from build123d import *

# Parameters (mm, degrees)
BOSS_EXTRUDE1_DEPTH      = 15
BOSS_EXTRUDE1_DEPTH_BACK = 15
SKETCH1_R                = 8.5
BOSS_EXTRUDE2_DEPTH      = 4
BOSS_EXTRUDE2_DEPTH_BACK = 4
FILLET1_R                = 5
SKETCH3_W                = 8
SKETCH3_H                = 8
BOSS_EXTRUDE3_DEPTH      = 17
BOSS_EXTRUDE4_DEPTH      = 6
BOSS_EXTRUDE4_DEPTH_BACK = 36
SKETCH4_R                = 3.5


with BuildPart() as part:
    # Sketch1 → Boss-Extrude1 (new, two sides: drawn at the far end of the back side and taken through both)
    with BuildSketch(Plane.XY.offset(-BOSS_EXTRUDE1_DEPTH_BACK)):
        Circle(SKETCH1_R)
    extrude(amount=BOSS_EXTRUDE1_DEPTH + BOSS_EXTRUDE1_DEPTH_BACK)

    # Sketch2 → Boss-Extrude2 (add, two sides: drawn at the far end of the back side and taken through both)
    with BuildSketch(Plane.XY.offset(-BOSS_EXTRUDE2_DEPTH_BACK)):
        with BuildLine():
            Line((-5, 6.873863542), (-5, 30))
            Line((-5, 30), (5, 30))
            Line((5, 30), (5, 6.873863542))
            ThreePointArc((5, 6.873863542), (0, 8.5), (-5, 6.873863542))
        make_face()
    extrude(amount=BOSS_EXTRUDE2_DEPTH + BOSS_EXTRUDE2_DEPTH_BACK)

    # Fillet1
    fillet1_edges = [part.edges().sort_by_distance(p)[0] for p in [
        (5, 6.873863542, 0),
        (0, 8.5, -4),
        (-5, 6.873863542, 0),
        (0, 8.5, 4),
    ]]
    fillet(fillet1_edges, radius=FILLET1_R)

    # Sketch3 → Boss-Extrude3 (add)
    with BuildSketch(Plane.ZY.offset(5)):
        with Locations((0, 26)):
            Rectangle(SKETCH3_W, SKETCH3_H)
    extrude(amount=BOSS_EXTRUDE3_DEPTH)

    # Sketch4 → Boss-Extrude4 (add, two sides: drawn at the far end of the back side and taken through both)
    with BuildSketch(Plane.XY.offset(15).offset(-BOSS_EXTRUDE4_DEPTH_BACK)):
        Circle(SKETCH4_R)
    extrude(amount=BOSS_EXTRUDE4_DEPTH + BOSS_EXTRUDE4_DEPTH_BACK)


solid = part.part
The model under review builds one solid part; all positions refer to its coordinate system, in mm. A direction names the side the tool comes from. Round coordinates to 2 decimals unless told otherwise and drop trailing zeros. Loops run counter-clockwise (first coordinate to the right, second up) from the corner with the lowest first, then second, coordinate; pieces in that order, holes last. Notation, with made-up numbers: M 63,77.25 L 76,77.25 A15 cw 76,91.25 Z; hole C -29.75,81 d3. An arc over 180 degrees is marked long. Answer as a JSON object with one key per item and string values.
Item 1: We need section C-C, the plane z = -3. State the section outline as (x, y) points, and give its area (3 significant figures).
Check sheet entries:
{"outline": "M -22,22 L -5,22 L -5,9.07 A5 cw -6.3,5.71 A8.5 ccw long 6.3,5.71 A5 cw 5,9.07 L 5,30 L -22,30 Z", "area": "584 mm2"}
Item 2: The part is to be moulded in two halves that separate along Y. For faces 4 (the face through (3.233, -1.341, -18.042)), 5 (the face through (5.345, 7.245, 0.126)), 6 (the face through (-5, 15, 0)), say which applies: +Y half, -Y half, draft (parallel to the pull), parting line (faces both ways), or undercut.
Check sheet entries:
{"face 4": "parting line", "face 5": "+Y half", "face 6": "undercut"}
Item 3: For line 1 along Z through (x, y) = (-14.5, 25); line 2 along Z through (x, y) = (5, 2); line 3 along X through (y, z) = (3, 10.5), list the stretches that pass through material, from the lowest coordinate up.
Check sheet entries:
{"line 1": "-4 to 4", "line 2": "-15 to 15", "line 3": "-7.95 to 7.95"}
Item 4: Clearance check with flat-ended pins moving along their axes: P1, Ø10, axis at x = 1.5, y = 22, coming from the -Z side; P2, Ø8, axis at y = 20.5, z = -9, coming from the -X side; P3, Ø5, axis at y = 14.5, z = 1, coming from the +X side; P4, Ø14, axis at x = -10, y = 19, coming from the +Z side. State where each tip first meets the part, or that it passes through.
Check sheet entries:
{"P1": "z = -4", "P2": "through", "P3": "x = 5", "P4": "z = 4"}
Item 5: We need section D-D, the plane x = -18. State the section outline as (y, z) points, and give its area (3 significant figures).
Check sheet entries:
{"outline": "M 22,-4 L 30,-4 L 30,4 L 22,4 Z", "area": "64.0 mm2"}
Item 6: We need section B-B, the plane x = 0. State the section outline as (y, z) points, and give its area (3 significant figures).
Check sheet entries:
{"outline": "M -8.5,-15 L -3.5,-15 L -3.5,-21 L 3.5,-21 L 3.5,-15 L 8.5,-15 L 8.5,-9 A5 cw 13.5,-4 L 30,-4 L 30,4 L 13.5,4 A5 cw 8.5,9 L 8.5,15 L 3.5,15 L 3.5,21 L -3.5,21 L -3.5,15 L -8.5,15 Z", "area": "777 mm2"}
Item 7: Tool access review of faces 1 (the face through (4, 0, -15)), 2 (the face through (-5.345, 7.245, 0.126)), 3 (the face through (5, 20, 0)): name each direction out of +Z, -Z, +X, -X, +Y, -Y from which nothing blocks a thin tool from reaching the whole face with its end or side.
Check sheet entries:
{"face 1": "-Z", "face 2": "+Z, -Z, -X", "face 3": "+Z, -Z, +X, +Y"}
Item 8: We need section A-A, the plane y = 0. State the section outline as (x, z) points, and give its area (3 significant figures).
Check sheet entries:
{"outline": "M -8.5,-15 L -3.5,-15 L -3.5,-21 L 3.5,-21 L 3.5,-15 L 8.5,-15 L 8.5,15 L 3.5,15 L 3.5,21 L -3.5,21 L -3.5,15 L -8.5,15 Z", "area": "594 mm2"}
